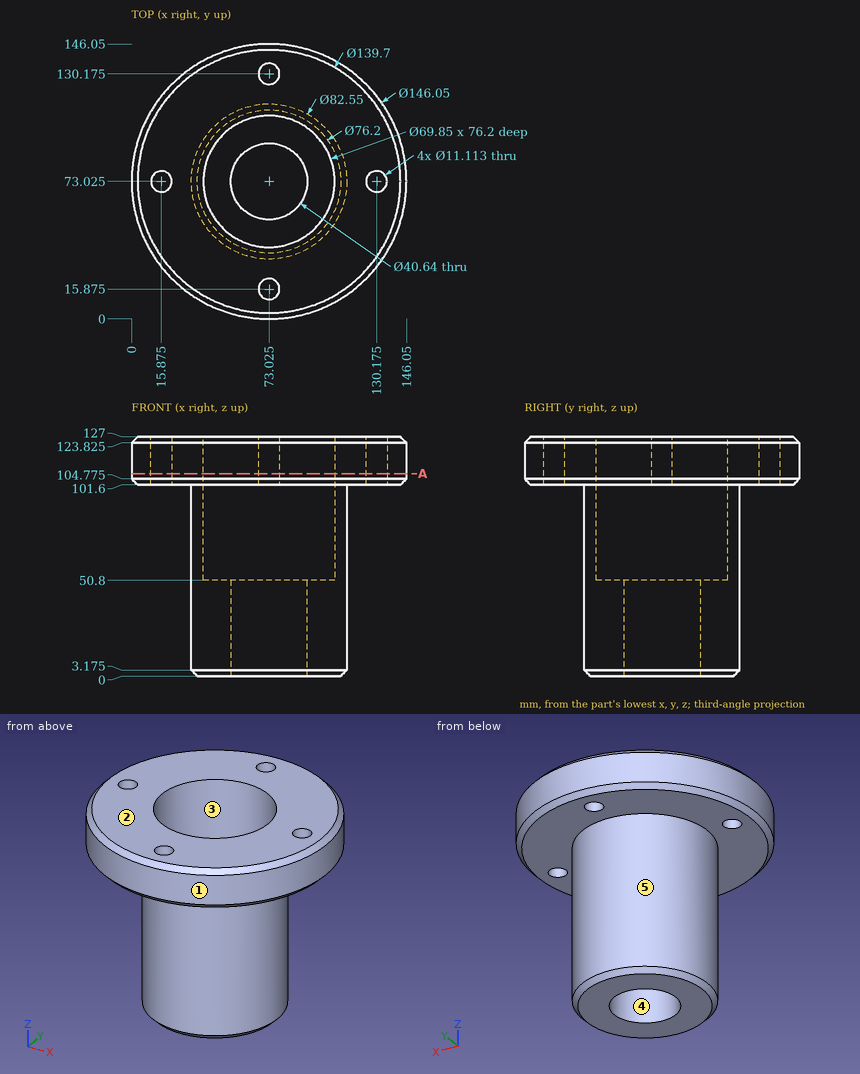
Geometry check sheet. Reference: drawing and pictorial views, mm from the part's lowest x, y, z. A direction names the side the tool comes from. Round coordinates to 2 decimals unless told otherwise and drop trailing zeros. Return JSON: item names as keys, results as strings. Group by question number.
(1) Set-up check for the marked faces 4 and 5: record each of +Z, -Z, +X, -X, +Y, -Y from which the full face is reachable in a straight line by a thin tool's end or side.
(2) Go/stop test with flat-tipped pins: pin 1 (18 mm diameter, centred on x = 73.025, y = 15.875, fed in from -Z); pin 2 (12 mm diameter, centred on y = 77.5, z = 91, fed in from +X); pin 3 (1.5 mm diameter, centred on y = 58, z = 36.5, fed in from +X). Record where each tip stops, or that it passes through.
(3) Scan lines: line 1 along Z through (x, y) = (129, 111.5); line 2 along X through (y, z) = (52, 68) (1 decimal); line 3 along X through (y, z) = (65.5, 112.5). Record each from-to range of solid material in increasing order. Write a range as [from, to].
(4) Section check A-A, the plane z = 107.5. Give the number of separate pieces and of enclosed holes in the cut face, and give its area (3 significant figures).
(5) Mould release check, pull along Y, two halves, no side actions. Record for the marked faces 1, 2 and 3: pulls with the +Y half, pulls with the -Y half, needs draft (parallel to the pull), parting line crosses it, or undercut.
Data:
{
 "1": {"face 4": "+Z, -Z", "face 5": "-Z"},
 "2": {"pin 1": "z = 101.6", "pin 2": "x = 114.3", "pin 3": "x = 111.75"},
 "3": {"line 1": "[101.6, 127]", "line 2": "[37.5, 45.1], [100.9, 108.5]", "line 3": "[0.39, 38.92], [107.13, 145.66]"},
 "4": {"separate pieces": "1", "enclosed holes": "5", "area": "12,500 mm²"},
 "5": {"face 1": "parting line crosses it", "face 2": "needs draft", "face 3": "undercut"}
}
